Build history of the part. All positions in model axes, mm. A direction names the side the tool comes from. Round coordinates to 2 decimals unless told otherwise and drop trailing zeros. Loops run counter-clockwise (first coordinate to the right, second up) from the corner with the lowest first, then second, coordinate; pieces in that order, holes last. Notation, with made-up numbers: (13.5, 27) - (56.5, 27) arc R8 cw to (56.5, 37) - close; hole circle Ø2 at (45, 21). An arc over 180 degrees is marked (long way). Use a Markdown table: item, result.
from build123d import *

# Parameters (mm, degrees)
SKETCH1_W           = 100
SKETCH1_H           = 90
SKETCH1_R           = 13.5
SKETCH1_R_2         = 2.65
SKETCH1_R_3         = 1.65
SKETCH1_R_4         = 2.25
BOSS_EXTRUDE1_DEPTH = 6
BOSS_EXTRUDE2_DEPTH = 8
SKETCH3_W           = 100
SKETCH3_H           = 6
BOSS_EXTRUDE3_DEPTH = 30
CUT_EXTRUDE1_REACH  = 106.173
SKETCH7_R           = 2.25
CUT_EXTRUDE2_DEPTH  = 3.5
BOSS_EXTRUDE4_DEPTH = 6


with BuildPart() as part:
    # Sketch1 → Boss-Extrude1 (new body)
    with BuildSketch(Plane(origin=(0, 0, 0), x_dir=(1, 0, 0), z_dir=(0, 1, 0))):
        Rectangle(SKETCH1_W, SKETCH1_H)
        with Locations(Location((0, 0, 0), (0, 0, 270))):
            Circle(SKETCH1_R, mode=Mode.SUBTRACT)
        with Locations(Location((0, 21.5, 0), (0, 0, 270))):
            Circle(SKETCH1_R_2, mode=Mode.SUBTRACT)
        with Locations(Location((23.0125, 0, 0), (0, 0, 270))):
            Circle(SKETCH1_R_3, mode=Mode.SUBTRACT)
        with Locations(Location((-23.0125, 0, 0), (0, 0, 270))):
            Circle(SKETCH1_R_3, mode=Mode.SUBTRACT)
        with Locations(Location((18.619546181, -10.75, 0), (0, 0, 270))):
            Circle(SKETCH1_R_2, mode=Mode.SUBTRACT)
        with Locations(Location((-18.619546181, -10.75, 0), (0, 0, 270))):
            Circle(SKETCH1_R_2, mode=Mode.SUBTRACT)
        with Locations(Location((-45, -40, 0), (0, 0, 270))):
            Circle(SKETCH1_R_4, mode=Mode.SUBTRACT)
        with Locations(Location((-45, 32.5, 0), (0, 0, 270))):
            Circle(SKETCH1_R_4, mode=Mode.SUBTRACT)
        with Locations(Location((45, 32.5, 0), (0, 0, 90))):
            Circle(SKETCH1_R_4, mode=Mode.SUBTRACT)
        with Locations(Location((45, -40, 0), (0, 0, 90))):
            Circle(SKETCH1_R_4, mode=Mode.SUBTRACT)
    extrude(amount=BOSS_EXTRUDE1_DEPTH)

    # Sketch2 → Boss-Extrude2 (add)
    with BuildSketch(Plane(origin=(0, 6, 0), x_dir=(1, 0, 0), z_dir=(0, 1, 0))):
        with BuildLine():
            Line((-30.2, 0), (-33.2, 0))
            Line((-33.2, 0), (-33.2, 39))
            Line((-33.2, 39), (33.2, 39))
            Line((33.2, 39), (33.2, 0))
            Line((33.2, 0), (30.2, 0))
            ThreePointArc((30.2, 0), (0, 30.2), (-30.2, 0))
        make_face()
    extrude(amount=BOSS_EXTRUDE2_DEPTH)

    # Sketch3 → Boss-Extrude3 (add)
    with BuildSketch(Plane(origin=(0, 6, 0), x_dir=(1, 0, 0), z_dir=(0, 1, 0))):
        with Locations((0, 42)):
            Rectangle(SKETCH3_W, SKETCH3_H)
    extrude(amount=BOSS_EXTRUDE3_DEPTH)

    # Sketch7 → Cut-Extrude1 (cut, up to next)
    with BuildSketch(Plane.XY.offset(-39), mode=Mode.PRIVATE) as cut_extrude1_sk1:
        with Locations((-45, 11)):
            Circle(SKETCH7_R)
    cut_extrude1_tool1 = extrude(cut_extrude1_sk1.sketch, amount=-CUT_EXTRUDE1_REACH, mode=Mode.PRIVATE) & part.part
    # Sketch7 → Cut-Extrude1 (cut, up to next)
    with BuildSketch(Plane.XY.offset(-39), mode=Mode.PRIVATE) as cut_extrude1_sk2:
        with Locations((45, 11)):
            Circle(SKETCH7_R)
    cut_extrude1_tool2 = extrude(cut_extrude1_sk2.sketch, amount=-CUT_EXTRUDE1_REACH, mode=Mode.PRIVATE) & part.part
    add(cut_extrude1_tool1.solids().sort_by_distance((-45, 11, -39))[0], mode=Mode.SUBTRACT)
    add(cut_extrude1_tool2.solids().sort_by_distance((45, 11, -39))[0], mode=Mode.SUBTRACT)

    # Sketch8 → Cut-Extrude2 (cut)
    with BuildSketch(Plane(origin=(0, 6, 0), x_dir=(1, 0, 0), z_dir=(0, 1, 0))):
        Polygon((19.548398385, 0), (21.280449192, -3), (24.744550808, -3), (26.476601615, 0), (24.744550808, 3), (21.280449192, 3), align=None)
        Polygon((-19.548398385, 0), (-21.280449192, 3), (-24.744550808, 3), (-26.476601615, 0), (-24.744550808, -3), (-21.280449192, -3), align=None)
    extrude(amount=-CUT_EXTRUDE2_DEPTH, mode=Mode.SUBTRACT)

    # Sketch9 → Boss-Extrude4 (add)
    with BuildSketch(Plane.ZY.offset(33.2)):
        Polygon((-39, 6), (-39, 31), (0, 6), align=None)
    boss_extrude4 = extrude(amount=BOSS_EXTRUDE4_DEPTH)

    # Mirror1: Boss-Extrude4 across plane
    add(boss_extrude4.mirror(Plane(origin=(0, 0, 0), x_dir=(0, 0, 1), z_dir=(1, 0, 0))))


solid = part.part
Q1. Pull direction Z, two halves, no side cores. Call faces 1 (the face through (21.247, 2.958, 10.405)), 2 (the face through (10, 0, -11)), 3 (the face through (25, 2.5, -1)), 4 (the face through (-1, 3, 45)): pulls with the +Z half, pulls with the -Z half, needs draft (parallel to the pull), parting line crosses it, or undercut.
Results found:
| item | result |
|---|---|
| face 1 | undercut |
| face 2 | needs draft |
| face 3 | undercut |
| face 4 | pulls with the +Z half |
Q2. Probe line 1 (X direction, y = 2, z = 0); line 2 (X direction, y = 1.7, z = -32.5); line 3 (X direction, y = 20, z = -24). List the from-to ranges inside material, lowest first.
Results found:
| item | result |
|---|---|
| line 1 | x = -50 to -24.66, -21.36 to -13.5, 13.5 to 21.36, 24.66 to 50 |
| line 2 | x = -50 to -47.25, -42.75 to 42.75, 47.25 to 50 |
| line 3 | x = -39.2 to -33.2, 33.2 to 39.2 |
Q3. Cut at C-C, the plane x = 0. List the corners of the cut face in (y, z).
Results found:
| item | result |
|---|---|
| outline | (0, -45) - (36, -45) - (36, -39) - (14, -39) - (14, -30.2) - (6, -30.2) - (6, -24.15) - (0, -24.15) - close; (0, -18.85) - (6, -18.85) - (6, -13.5) - (0, -13.5) - close; (0, 13.5) - (6, 13.5) - (6, 45) - (0, 45) - close |
Q4. Which spindle directions (+Z, -Z, +X, -X, +Y, -Y) get a long thin tool onto all of the face, cutting with end or side? Do faces 5 (the face through (-12, 6, 12)), 6 (the face through (50, 5, -13)), 7 (the face through (36.158, 18.675, -19.773)), 8 (the face through (-43.103, 2.958, -31.29)), 9 (the face through (25.62, 4.27, -1.48)). Say none if no direction does.
Results found:
| item | result |
|---|---|
| face 5 | +Z, +Y |
| face 6 | +Z, -Z, +X, +Y, -Y |
| face 7 | +Z, +X, +Y |
| face 8 | +Y, -Y |
| face 9 | +Y |
Q5. Cut at A-A, the plane y = 11. List the corners of the cut face in (x, z), plus the area to 3 significant figures.
Results found:
| item | result |
|---|---|
| outline | (-50, -45) - (-47.25, -45) - (-47.25, -39) - (-50, -39) - close; (-42.75, -45) - (42.75, -45) - (42.75, -39) - (39.2, -39) - (39.2, -7.8) - (33.2, -7.8) - (33.2, 0) - (30.2, 0) arc R30.2 cw to (-30.2, 0) - (-33.2, 0) - (-33.2, -7.8) - (-39.2, -7.8) - (-39.2, -39) - (-42.75, -39) - close; (47.25, -45) - (50, -45) - (50, -39) - (47.25, -39) - close |
| area | 2,080 mm2 |
Q6. Cut at D-D, the plane x = -45. List the corners of the cut face in (y, z), plus the area to 3 significant figures.
Results found:
| item | result |
|---|---|
| outline | (0, -45) - (8.75, -45) - (8.75, -39) - (6, -39) - (6, -34.75) - (0, -34.75) - close; (0, -30.25) - (6, -30.25) - (6, 37.75) - (0, 37.75) - close; (0, 42.25) - (6, 42.25) - (6, 45) - (0, 45) - close; (13.25, -45) - (36, -45) - (36, -39) - (13.25, -39) - close |
| area | 639 mm2 |
Q7. Cut at B-B, the plane z = 40. List the corners of the cut face in (x, y).
Results found:
| item | result |
|---|---|
| outline | (-50, 0) - (-47.25, 0) - (-47.25, 6) - (-50, 6) - close; (-42.75, 0) - (42.75, 0) - (42.75, 6) - (-42.75, 6) - close; (47.25, 0) - (50, 0) - (50, 6) - (47.25, 6) - close |
Q8. Drop flat-ended pins along their axis: pin 1 (2 mm diameter, centred on x = 38, z = 9, fed in from +Y); pin 2 (7 mm diameter, centred on x = 45, z = 40, fed in from -Y); pin 3 (2.5 mm diameter, centred on y = 8.5, z = -5.5, fed in from +X); pin 4 (1.5 mm diameter, centred on x = 31.5, y = 8, fed in from +Z). Give the stop position or say it passes through.
Results found:
| item | result |
|---|---|
| pin 1 | stops at y = 6 |
| pin 2 | stops at y = 0 |
| pin 3 | stops at x = 39.2 |
| pin 4 | stops at z = 0 |
